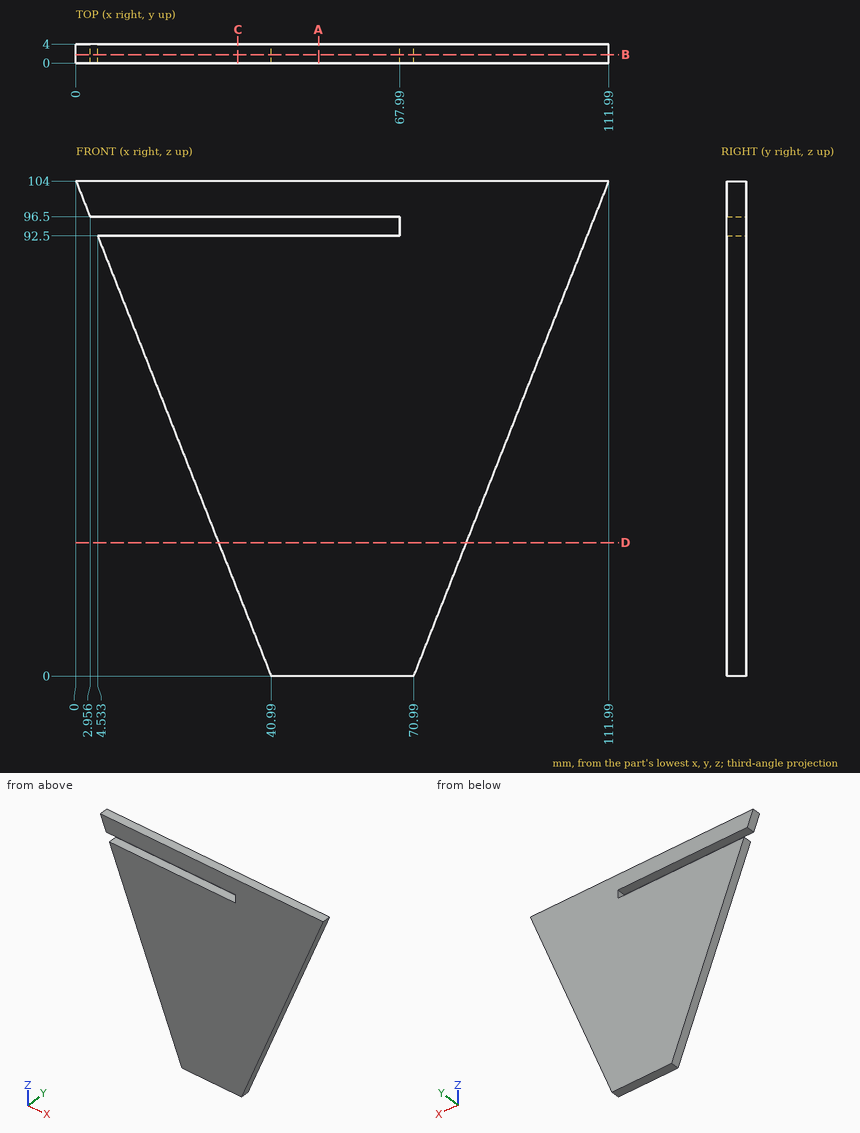
Study the drawing (mm; zero at the part's minimum x, y, z) and answer. Coordinates: 2 decimals unless noted, no trailing zeros. Loops run counter-clockwise (first coordinate to the right, second up) from the corner with the lowest first, then second, coordinate; pieces in that order, holes last. Notation, with made-up numbers: M -5.75,-2.5 L 39.25,-2.5 A26 ccw 39.25,13.5 Z; hole C 39.25,66 d7. An arc over 180 degrees is marked long. Answer as a JSON object with one key per item and string values. Group by question number.
Item 1: Consider L1, parallel to Z at x = 61, y = 0.9; L2, parallel to X at y = 3.85, z = 78.5; L3, parallel to X at y = 1.7, z = 16 (1 decimal). Determine where each line is inside the solid, lowest interval first.
Item 2: Section B-B (y = 1.75) is taken. Write down the section's boundary in (x, z), and give its area (3 significant figures).
Item 3: Section C-C (x = 34) is taken. Write down the section's boundary in (y, z) (1 decimal), and give its area (3 significant figures).
Item 4: Section D-D (z = 28) is taken. Write down the section's boundary in (x, y) (1 decimal).
Item 5: Section A-A (x = 51) is taken. Write down the section's boundary in (y, z).
Solved:
{
 "1": {"L1": "z = 0 to 92.5, 96.5 to 104", "L2": "x = 10.05 to 101.94", "L3": "x = 34.7 to 77.3"},
 "2": {"outline": "M 0,104 L 2.96,96.5 L 67.99,96.5 L 67.99,92.5 L 4.53,92.5 L 40.99,0 L 70.99,0 L 111.99,104 Z", "area": "7,130 mm2"},
 "3": {"outline": "M 0,17.7 L 4,17.7 L 4,92.5 L 0,92.5 Z; M 0,96.5 L 4,96.5 L 4,104 L 0,104 Z", "area": "329 mm2"},
 "4": {"outline": "M 30,0 L 82,0 L 82,4 L 30,4 Z"},
 "5": {"outline": "M 0,0 L 4,0 L 4,92.5 L 0,92.5 Z; M 0,96.5 L 4,96.5 L 4,104 L 0,104 Z"}
}
